Work out the finished part from the listing and answer in its coordinate system (mm). A direction names the side the tool comes from. Coordinates: 2 decimals unless noted, no trailing zeros. Write each loop counter-clockwise with the first axis right and the second up, starting at its lowest first coordinate (ties: lowest second). Pieces come first, ordered by that corner, then holes. Notation, with made-up numbers: (74, -20.75) -> (106, -20.75) arc R13 ccw to (106, -6.75) -> close; hole circle Ø9 at (-26, 55). An arc over 180 degrees is marked (long way). Write each question's results on one line, items separated by ' | '. Start each with the question number.
Autodesk Inventor part; units mm, degrees
ref_plane "YZ Plane" through (0, 0, 0) normal (1, 0, 0) x (0, 1, 0)
ref_plane "XZ Plane" through (0, 0, 0) normal (0, 1, 0) x (-1, 0, 0)
ref_plane "XY Plane" through (0, 0, 0) normal (0, 0, 1) x (1, 0, 0)
sketch "Sketch1" plane through (0, 0, 0) normal (0, 1, 0) x (-1, 0, 0)
  line L0 (0, 0) -> (5.08, 0)
  line L1 (5.08, 0) -> (5.08, 3.81)
  line L2 (2.54, 6.35) -> (0, 6.35)
  line L3 (0, 6.35) -> (0, 0)
  arc A0 (5.08, 3.81) -> (2.54, 6.35) centre (2.54, 3.81) ccw
  line L4 (1.5875, 0) -> (1.5875, 1.27)
  line L5 (1.5875, 1.27) -> (2.2294, 1.27)
  line L6 (2.2294, 1.27) -> (2.2294, 6.35)
  dimension "d0" = 2.54
  dimension "d1" = 5.08
  dimension "d2" = 6.35
  dimension "d3" = 1.5875
  dimension "d5" = 1.27
revolve "Revolution1" add sketch "Sketch1" angle 360 about axis through (0, 0, 6.35) along (0, 0, -1) contours L4 L5 L6 L2 A0 L1 L0
properties part number "Feet"
1. Find the intervals of material crossed by L1, parallel to Y at x = 0, z = 3.25; L2, parallel to X at y = 0.75, z = 0.5; L3, parallel to X at y = -1, z = 4, in increasing order.
2. Given pin 1 Ø1 at (y, z) = (2.5, 2) entering from -X; pin 2 Ø1 at (x, y) = (3.5, -4) entering from +Z; pin 3 Ø1.5 at (y, z) = (-1.5, 5) entering from +X, each flat-ended and moving along its own axis, determine where each tip first touches the part or whether it passes through.
3. Find section A-A on z = 1.5. Give the vertices of the cut face in (x, y), and give its area (3 significant figures).
4. Determine the mould class of faces 1 (the face through (-2, 0, 0)), 2 (the face through (0.661, -5.037, 1.932)), 3 (the face through (-1.5, -1, 1.27)) for opening direction X: pulls with the +X half, pulls with the -X half, needs draft (parallel to the pull), parting line crosses it, or undercut.
5. For faces 4 (the face through (0.34, 1.55, 0.64)), 5 (the face through (0.29, -2.21, 3.85)), determine the directions among +Z, -Z, +X, -X, +Y, -Y from which every point of the face is accessible in a straight line to the end or side of a thin tool.
Ans:
1) L1: y = -5.08 to -2.23, 2.23 to 5.08 | L2: x = -5.02 to -1.4, 1.4 to 5.02 | L3: x = -4.97 to -1.99, 1.99 to 4.97
2) pin 1: stops at x = -4.67 | pin 2: stops at z = 4.94 | pin 3: stops at x = 4.9
3) outline: circle Ø10.16 at (0, 0); hole circle Ø4.46 at (0, 0) | area: 65.5 mm²
4) face 1: needs draft | face 2: parting line crosses it | face 3: undercut
5) face 4: +Z, -Z | face 5: +Z
